CAD build for the part. Positions are in the model's coordinates, mm. Face numbers are marked on the shaded views. A direction names the side the tool comes from. Coordinates: 2 decimals unless noted, no trailing zeros. Order: outer loops, then holes, each group sorted by start corner. A loop starts at its lowest first (then second) coordinate and runs counter-clockwise, first axis right, second up. Notation, with made-up numbers: (-19, 71.25) - (13, 71.25) arc R6 ccw to (13, 79.25) - close; hole circle Ø11 at (64.25, 52). An arc over 180 degrees is marked (long way). Return JSON: item names as keys, results as strings.
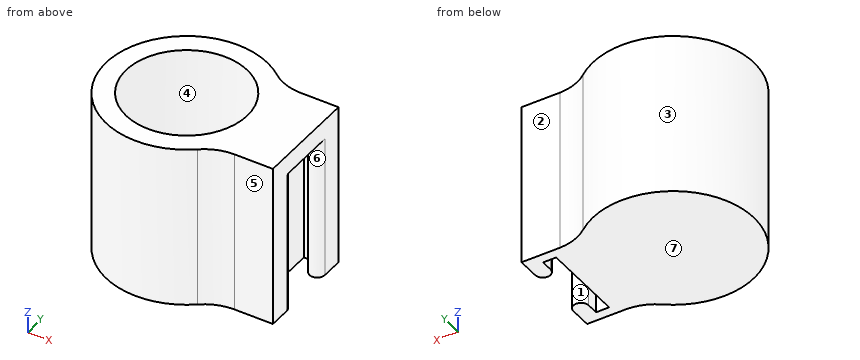
from build123d import *

# Parameters (mm, degrees)
F0_R     = 9.652
F1_DEPTH = 22.86
F2_R     = 9.652
F3_DEPTH = 3.175
F4_R     = 9.652
F5_DEPTH = 3.175


with BuildPart() as f1:
    # F0 (on Top) → F1 (new body)
    with BuildSketch(Plane.XY):
        with BuildLine():
            Line((14.4724995292, -6.4216016291), (14.4724995292, 6.2783983709))
            Line((14.4724995292, 6.2783983709), (14.4724995292, 6.6347159585))
            Line((14.4724995292, 6.6347159585), (14.5994995292, 6.6347159585))
            Line((14.5994995292, 6.6347159585), (16.1869995292, 6.6347159585))
            Line((16.1869995292, 6.6347159585), (16.5567258399, 6.6347159585))
            Line((16.5567258399, 6.6347159585), (16.5567258399, 4.7932159585))
            ThreePointArc((16.5567258399, 4.7932159585), (17.7744995292, 3.5754422692), (18.9922732184, 4.7932159585))
            Line((18.9922732184, 4.7932159585), (18.9922732184, 6.6347159585))
            Line((18.9922732184, 6.6347159585), (18.9922732184, 8.2222159585))
            Line((18.9922732184, 8.2222159585), (14.4724995292, 8.2222159585))
            Line((14.4724995292, 8.2222159585), (12.8849995292, 8.2222159585))
            ThreePointArc((12.8849995292, 8.2222159585), (10.3328098948, 8.6905993264), (8.0737784074, 9.9672479265))
            ThreePointArc((8.0737784074, 9.9672479265), (-12.827, 0), (8.0737784074, -9.9672479265))
            ThreePointArc((8.0737784074, -9.9672479265), (10.3329433344, -8.7017229937), (12.8849995292, -8.2631016291))
            Line((12.8849995292, -8.2631016291), (14.4724995292, -8.2631016291))
            Line((14.4724995292, -8.2631016291), (18.9922732184, -8.2631016291))
            Line((18.9922732184, -8.2631016291), (18.9922732184, -6.6756016291))
            Line((18.9922732184, -6.6756016291), (18.9922732184, -4.8341016291))
            ThreePointArc((18.9922732184, -4.8341016291), (17.7744995292, -3.6163279398), (16.5567258399, -4.8341016291))
            Line((16.5567258399, -4.8341016291), (16.5567258399, -6.6756016291))
            Line((16.5567258399, -6.6756016291), (16.1869995292, -6.6756016291))
            Line((16.1869995292, -6.6756016291), (14.4724995292, -6.6756016291))
            Line((14.4724995292, -6.6756016291), (14.4724995292, -6.4216016291))
        make_face()
        Circle(F0_R, mode=Mode.SUBTRACT)
    extrude(amount=F1_DEPTH)

    # F2 (on face) → F3 (join)
    with BuildSketch(Plane.XY.offset(22.86)):
        with BuildLine():
            ThreePointArc((12.8849995292, 8.2222159585), (10.3328098948, 8.6905993264), (8.0737784074, 9.9672479265))
            ThreePointArc((8.0737784074, 9.9672479265), (-12.827, 0), (8.0737784074, -9.9672479265))
            ThreePointArc((8.0737784074, -9.9672479265), (10.3329433344, -8.7017229937), (12.8849995292, -8.2631016291))
            Line((12.8849995292, -8.2631016291), (18.9922732184, -8.2631016291))
            Line((18.9922732184, -8.2631016291), (18.9922732184, -4.8341016291))
            ThreePointArc((18.9922732184, -4.8341016291), (17.7744995292, -3.6163279398), (16.5567258399, -4.8341016291))
            Line((16.5567258399, -4.8341016291), (16.5567258399, -6.6756016291))
            Line((16.5567258399, -6.6756016291), (14.4724995292, -6.6756016291))
            Line((14.4724995292, -6.6756016291), (14.4724995292, 6.6347159585))
            Line((14.4724995292, 6.6347159585), (16.5567258399, 6.6347159585))
            Line((16.5567258399, 6.6347159585), (16.5567258399, 4.7932159585))
            ThreePointArc((16.5567258399, 4.7932159585), (17.7744995292, 3.5754422692), (18.9922732184, 4.7932159585))
            Line((18.9922732184, 4.7932159585), (18.9922732184, 8.2222159585))
            Line((18.9922732184, 8.2222159585), (12.8849995292, 8.2222159585))
        make_face()
        Circle(F2_R, mode=Mode.SUBTRACT)
        with BuildLine():
            Line((18.9922732184, -4.8341016291), (18.9922732184, 4.7932159585))
            ThreePointArc((18.9922732184, 4.7932159585), (17.7744995292, 3.5754422692), (16.5567258399, 4.7932159585))
            Line((16.5567258399, 4.7932159585), (16.5567258399, 6.6347159585))
            Line((16.5567258399, 6.6347159585), (14.4724995292, 6.6347159585))
            Line((14.4724995292, 6.6347159585), (14.4724995292, -6.6756016291))
            Line((14.4724995292, -6.6756016291), (16.5567258399, -6.6756016291))
            Line((16.5567258399, -6.6756016291), (16.5567258399, -4.8341016291))
            ThreePointArc((16.5567258399, -4.8341016291), (17.7744995292, -3.6163279398), (18.9922732184, -4.8341016291))
        make_face()
    extrude(amount=F3_DEPTH)

    # F4 (on face) → F5 (join)
    with BuildSketch(Plane(origin=(0, 0, 0), x_dir=(1, 0, 0), z_dir=(0, 0, -1))):
        with BuildLine():
            Line((18.9922732184, 8.2631016291), (12.8849995292, 8.2631016291))
            ThreePointArc((12.8849995292, 8.2631016291), (10.3329433344, 8.7017229937), (8.0737784074, 9.9672479265))
            ThreePointArc((8.0737784074, 9.9672479265), (-12.827, 0), (8.0737784074, -9.9672479265))
            ThreePointArc((8.0737784074, -9.9672479265), (10.3328098948, -8.6905993264), (12.8849995292, -8.2222159585))
            Line((12.8849995292, -8.2222159585), (18.9922732184, -8.2222159585))
            Line((18.9922732184, -8.2222159585), (18.9922732184, -4.7932159585))
            ThreePointArc((18.9922732184, -4.7932159585), (17.7744995292, -3.5754422692), (16.5567258399, -4.7932159585))
            Line((16.5567258399, -4.7932159585), (16.5567258399, -6.6347159585))
            Line((16.5567258399, -6.6347159585), (14.4724995292, -6.6347159585))
            Line((14.4724995292, -6.6347159585), (14.4724995292, 6.6756016291))
            Line((14.4724995292, 6.6756016291), (16.5567258399, 6.6756016291))
            Line((16.5567258399, 6.6756016291), (16.5567258399, 4.8341016291))
            ThreePointArc((16.5567258399, 4.8341016291), (17.7744995292, 3.6163279398), (18.9922732184, 4.8341016291))
            Line((18.9922732184, 4.8341016291), (18.9922732184, 8.2631016291))
        make_face()
        Circle(F4_R, mode=Mode.SUBTRACT)
        Circle(F4_R)
    extrude(amount=-F5_DEPTH)


solid = f1.part
Item 1: Band-saw the part on A-A, the plane z = 2.5. List the corners of the cut face in (x, y) (1 decimal).
Findings below:
{"outline": "(8.1, -10) arc R7.6 cw to (12.9, -8.3) - (19, -8.3) - (19, -4.8) arc R1.2 ccw to (16.6, -4.8) - (16.6, -6.7) - (14.5, -6.7) - (14.5, 6.6) - (16.6, 6.6) - (16.6, 4.8) arc R1.2 ccw to (19, 4.8) - (19, 8.2) - (12.9, 8.2) arc R7.8 cw to (8.1, 10) arc R12.8 ccw (long way) to start"}
Item 2: Drop flat-ended pins along their axis: P1, Ø4, axis at y = -8.5, z = 21.5, coming from the -X side; P2, Ø4, axis at x = 2, z = 20.5, coming from the +Y side; P3, Ø5, axis at x = 15.5, z = 15.5, coming from the -Y side; P4, Ø0.9, axis at y = 6, z = 12, coming from the -X side. Give the stop position or say it passes through.
Findings below:
{"P1": "stops at x = -11.06", "P2": "stops at y = 12.83", "P3": "stops at y = -8.26", "P4": "stops at x = -11.56"}
Item 3: Band-saw the part on B-B, the plane x = 0. List the corners of the cut face in (y, z) (3 decimals).
Findings below:
{"outline": "(-12.827, 0) - (12.827, 0) - (12.827, 26.035) - (9.652, 26.035) - (9.652, 3.175) - (-9.652, 3.175) - (-9.652, 26.035) - (-12.827, 26.035) - close"}
Item 4: Band-saw the part on C-C, the plane y = 0. List the corners of the cut face in (x, z) (1 decimal).
Findings below:
{"outline": "(-12.8, 0) - (14.5, 0) - (14.5, 22.9) - (19, 22.9) - (19, 26) - (9.7, 26) - (9.7, 3.2) - (-9.7, 3.2) - (-9.7, 26) - (-12.8, 26) - close"}
Item 5: Band-saw the part on D-D, the plane y = -5.25. List the corners of the cut face in (x, z) (1 decimal), then the cut area to 3 significant figures.
Findings below:
{"outline": "(-11.7, 0) - (14.5, 0) - (14.5, 22.9) - (16.6, 22.9) - (16.6, 0) - (19, 0) - (19, 26) - (8.1, 26) - (8.1, 3.2) - (-8.1, 3.2) - (-8.1, 26) - (-11.7, 26) - close", "area": "381 mm²"}
Item 6: Mould opens along Y. For the marked faces 5, 6 and 7 say: released by +Y, released by -Y, zero draft, split by the parting line, or undercut.
Findings below:
{"face 5": "released by -Y", "face 6": "undercut", "face 7": "zero draft"}
Item 7: Wall check: L1, parallel to Y at x = 0, z = 13.25; L2, parallel to X at y = 0, z = 17.5; L3, parallel to X at y = 5.25, z = 20.25. Give the ranges that are in metal, low to high. Write a range as [from, to].
Findings below:
{"L1": "y = [-12.83, -9.65], [9.65, 12.83]", "L2": "x = [-12.83, -9.65], [9.65, 14.47]", "L3": "x = [-11.7, -8.1], [8.1, 14.47], [16.56, 18.99]"}
Item 8: Which spindle directions (+Z, -Z, +X, -X, +Y, -Y) get a long thin tool onto all of the face, cutting with end or side? Do the marked faces 1, 2, 3 and 4. Say none if no direction does.
Findings below:
{"face 1": "-Z", "face 2": "+Z, -Z, +X, +Y", "face 3": "+Z, -Z", "face 4": "+Z"}
